from build123d import *

# Parameters (mm, degrees)
F0_R     = 38.1
F1_DEPTH = 76.2
F2_R     = 12.7
F3_DEPTH = 12.7
F4_R     = 12.7
F5_DEPTH = 12.7


with BuildPart() as f1:
    # F0 (on Right) → F1 (new body)
    with BuildSketch(Plane.YZ):
        Circle(F0_R)
    extrude(amount=F1_DEPTH)

    # F2 (on face) → F3 (join)
    with BuildSketch(Plane(origin=(0, 0, 0), x_dir=(0, -1, 0), z_dir=(-1, 0, 0))):
        Circle(F2_R)
    extrude(amount=F3_DEPTH)

    # F4 (on face) → F5 (join)
    with BuildSketch(Plane.YZ.offset(76.2)):
        Circle(F4_R)
    extrude(amount=F5_DEPTH)


solid = f1.part
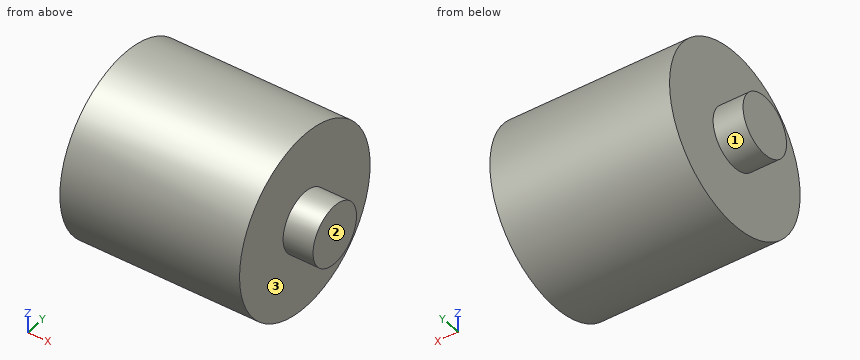
Could you check a few things on this model? Use its own coordinates, in mm. Face numbers are marked on the shaded views. A direction names the side the tool comes from. Coordinates: 2 decimals unless noted, no trailing zeros. Write each loop counter-clockwise with the first axis right and the second up, starting at its lowest first coordinate (ties: lowest second). Pieces come first, ordered by that corner, then holes. Notation, with made-up numbers: M 19.25,8.5 L 59.25,8.5 A31 ccw 59.25,35.5 Z; hole C 83.25,-14.75 d4. An arc over 180 degrees is marked long. One line per question, with ' | ' between items.
1) For pin 1 Ø2 at (x, y) = (48, 12.5) entering from +Z; pin 2 Ø5 at (y, z) = (23, -7) entering from -X; pin 3 Ø3 at (y, z) = (18.5, 24) entering from +X, each with a flat end and sliding along its axis, tell me the tip position at first contact or that it passes through.
Checks:
pin 1: z = 36.32 | pin 2: x = 0 | pin 3: x = 76.2
2) Imagine slicing it at A-A, the plane z = 0. Write out the boundary of the cut face in (x, y), and give its area (3 significant figures).
Checks:
outline: M -12.7,-12.7 L 0,-12.7 L 0,-38.1 L 76.2,-38.1 L 76.2,-12.7 L 88.9,-12.7 L 88.9,12.7 L 76.2,12.7 L 76.2,38.1 L 0,38.1 L 0,12.7 L -12.7,12.7 Z | area: 6,450 mm²
3) For the marked faces 1, 2 and 3, which set-ups out of +Z, -Z, +X, -X, +Y, -Y let a thin tool reach every point of the face, with its end or its side?
Checks:
face 1: -X | face 2: +Z, -Z, +X, +Y, -Y | face 3: +X
4) I need wall thicknesses on probe 1 along X at (y, z) = (-25, -25); probe 2 along Y at (x, z) = (10.5, 7.5); probe 3 along Y at (x, z) = (5, 22). Which ranges of each line are inside material? Lowest first, please. Write a range as [from, to].
Checks:
probe 1: [0, 76.2] | probe 2: [-37.35, 37.35] | probe 3: [-31.11, 31.11]
5) Imagine slicing it at D-D, the plane x = -1.5. Write out the boundary of the cut face in (y, z).
Checks:
outline: C 0,0 d25.4
6) Imagine slicing it at C-C, the plane x = 40.5. Write out the boundary of the cut face in (y, z), and give its area (3 significant figures).
Checks:
outline: C 0,0 d76.2 | area: 4,560 mm²
